from build123d import *

# Parameters (mm, degrees)
SKETCH1_W                = 8.5
SKETCH1_H                = 8.5
BOSS_EXTRUDE1_DEPTH      = 10
SKETCH2_W                = 7
SKETCH2_H                = 7
BOSS_EXTRUDE2_DEPTH      = 10.01
BOSS_EXTRUDE2_DEPTH_BACK = 0.01
FILLET2_R                = 0.5
SKETCH35_R               = 1.25
CUT_EXTRUDE1_DEPTH       = 20
SWEEP1_PROFILE_R         = 0.35


with BuildPart() as part:
    # Sketch1 → Boss-Extrude1 (new body)
    with BuildSketch(Plane(origin=(0, 0, 0), x_dir=(1, 0, 0), z_dir=(0, 1, 0))):
        Rectangle(SKETCH1_W, SKETCH1_H)
    extrude(amount=BOSS_EXTRUDE1_DEPTH)

    # Sketch2 → Boss-Extrude2 (add, two sides)
    with BuildSketch(Plane(origin=(0, 0, 0), x_dir=(1, 0, 0), z_dir=(0, 1, 0))) as boss_extrude2_sk:
        Rectangle(SKETCH2_W, SKETCH2_H)
    extrude(amount=BOSS_EXTRUDE2_DEPTH)
    extrude(boss_extrude2_sk.sketch, amount=-BOSS_EXTRUDE2_DEPTH_BACK)

    # Fillet2
    fillet2_edges = [part.edges().sort_by_distance(p)[0] for p in [
        (4.25, 5, 4.25),
        (-4.25, 5, 4.25),
        (-4.25, 5, -4.25),
        (4.25, 5, -4.25),
    ]]
    fillet(fillet2_edges, radius=FILLET2_R)

    # Sketch35 → Cut-Extrude1 (cut)
    with BuildSketch(Plane(origin=(0, 10.01, 0), x_dir=(1, 0, 0), z_dir=(0, 1, 0))):
        with Locations(Location((0, 0, 0), (0, 0, 270))):  # turned: the seam where the file's is
            Circle(SKETCH35_R)
    extrude(amount=-CUT_EXTRUDE1_DEPTH, mode=Mode.SUBTRACT)

    # Sweep1: sweep along a path in Sketch37
    with BuildLine(Plane.XY) as sweep1_path:
        Line((4.25, 7), (4.55, 7))
        ThreePointArc((4.55, 7), (4.903553391, 6.853553391), (5.05, 6.5))
        Line((5.05, 6.5), (5.05, -68.5))
    # Sweep1 profile (on start of the path) → Sweep1 (sweep)
    with BuildSketch(Plane(origin=(4.25, 7, 0), x_dir=(0, 0, 1), z_dir=(1, 0, 0))):
        Circle(SWEEP1_PROFILE_R)
    sweep1 = sweep(path=sweep1_path.line)

    # Mirror1: Sweep1 across plane
    add(sweep1.mirror(Plane(origin=(0, 0, 0), x_dir=(0, 0, 1), z_dir=(1, 0, 0))))


solid = part.part
Source: CAD feature listing. Evaluate the final solid. Frame: model axes, mm. Give positions to 0.01 mm unless a question says otherwise; leave off trailing zeros. Write each loop counter-clockwise with the first axis right and the second up, starting at its lowest first coordinate (ties: lowest second). Pieces come first, ordered by that corner, then holes. Notation, with made-up numbers: (-15.75, 78) -> (20.25, 78) arc R26 cw to (20.25, 95) -> close; hole circle Ø7 at (-8.75, 5.25). An arc over 180 degrees is marked (long way). Return JSON: item names as keys, results as strings. Group by question number.
1. Section C-C, the plane y = -30. Output: boundary loops of the cut face in (x, z).
2. Pin query (flat end, axial travel): pin 1 Ø3 at (x, z) = (-2, 1) entering from -Y. Return the tip coordinate at first contact, or that it passes through.
3. Mould query, pull axis X, two halves, no side actions, for faces 1 (the face through (-1.22, 5.07, -0.27)), 2 (the face through (-2, 10.01, 0)). Classes: +X half, -X half, draft (parallel to the pull), parting line (faces both ways), or undercut.
4. Material intervals for line 1 (X direction, y = 2.75, z = 0); line 2 (X direction, y = 7.75, z = 0); line 3 (Y direction, x = 4.5, z = 0), sorted ascending. Write a range as from..to.
Determined:
{
 "1": {"outline": "circle Ø0.7 at (-5.05, 0); circle Ø0.7 at (5.05, 0)"},
 "2": {"pin 1": "stops at y = -0.01"},
 "3": {"face 1": "undercut", "face 2": "draft"},
 "4": {"line 1": "x = -5.4..-4.7, -4.25..-1.25, 1.25..4.25, 4.7..5.4", "line 2": "x = -4.25..-1.25, 1.25..4.25", "line 3": "y = 6.65..7.35"}
}
